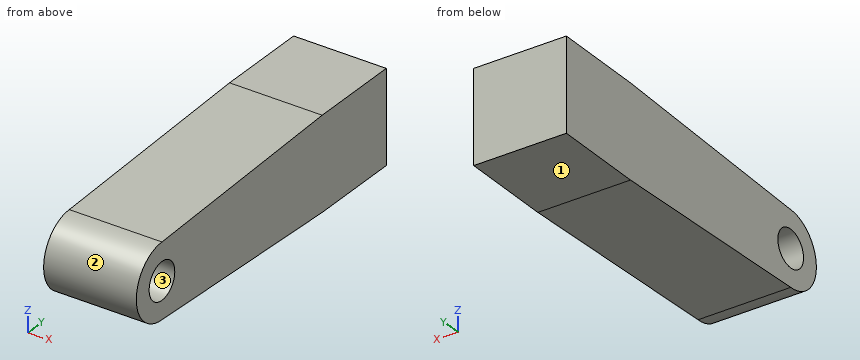
```python
from build123d import *

# Parameters (mm, degrees)
CROQUIS1_R              = 0.5
SALIENTE_EXTRUIR1_DEPTH = 2.5


with BuildPart() as part:
    # Croquis1 → Saliente-Extruir1 (new body)
    with BuildSketch(Plane(origin=(0, 0, 0), x_dir=(0, 0, -1), z_dir=(1, 0, 0))):
        with BuildLine():
            Line((1.25, 1.25), (-1.25, 1.25))
            Line((-1.25, 1.25), (-1.25, -1.25))
            Line((-1.25, -1.25), (-1, -7.5))
            ThreePointArc((-1, -7.5), (0, -8.5), (1, -7.5))
            Line((1, -7.5), (1.25, -1.25))
            Line((1.25, -1.25), (1.25, 1.25))
        make_face()
        with Locations((0, -7.5)):
            Circle(CROQUIS1_R, mode=Mode.SUBTRACT)
    extrude(amount=SALIENTE_EXTRUIR1_DEPTH)


solid = part.part
```
Can you work these out from the model? Positions are in its coordinate system, mm. Face numbers are marked on the shaded views. Coordinates: 2 decimals unless noted, no trailing zeros. Write each loop counter-clockwise with the first axis right and the second up, starting at its lowest first coordinate (ties: lowest second). Pieces come first, ordered by that corner, then holes. Notation, with made-up numbers: M 43.25,42.5 L 85.25,42.5 A18 ccw 85.25,47.5 Z; hole C 69.5,-7.5 d10. An arc over 180 degrees is marked long. Answer as CSV lines item,"result".
Item 1: Imagine slicing it at A-A on z = 0. List the corners of the cut face in (x, y) for me.
Geometry results:
outline,"M 0,-8.5 L 2.5,-8.5 L 2.5,-8 L 0,-8 Z; M 0,-7 L 2.5,-7 L 2.5,1.25 L 0,1.25 Z"
Item 2: Imagine slicing it at C-C on y = -5.5. List the corners of the cut face in (x, z) for me.
Geometry results:
outline,"M 0,-1.08 L 2.5,-1.08 L 2.5,1.08 L 0,1.08 Z"
Item 3: Imagine slicing it at B-B on x = 1.6. List the corners of the cut face in (y, z) for me.
Geometry results:
outline,"M -7.5,-1 L -1.25,-1.25 L 1.25,-1.25 L 1.25,1.25 L -1.25,1.25 L -7.5,1 A1 ccw Z; hole C -7.5,0 d1"
Item 4: We'd pull the mould along Y, two halves only. Please class the marked faces 1, 2 and 3: +Y half, -Y half, draft (parallel to the pull), parting line (faces both ways), or undercut.
Geometry results:
face 1,"draft"
face 2,"-Y half"
face 3,"undercut"
Item 5: Please list where these lines run through material, in increasing order: line 1 along Y through (x, z) = (0.9, 0); line 2 along Y through (x, z) = (1.65, 0.3); line 3 along Z through (x, y) = (2.2, -7.75).
Geometry results:
line 1,"y = -8.5 to -8, -7 to 1.25"
line 2,"y = -8.45 to -7.9, -7.1 to 1.25"
line 3,"z = -0.97 to -0.43, 0.43 to 0.97"
Item 6: Imagine slicing it at D-D on y = -2.75. List the corners of the cut face in (x, z) for me.
Geometry results:
outline,"M 0,-1.19 L 2.5,-1.19 L 2.5,1.19 L 0,1.19 Z"
